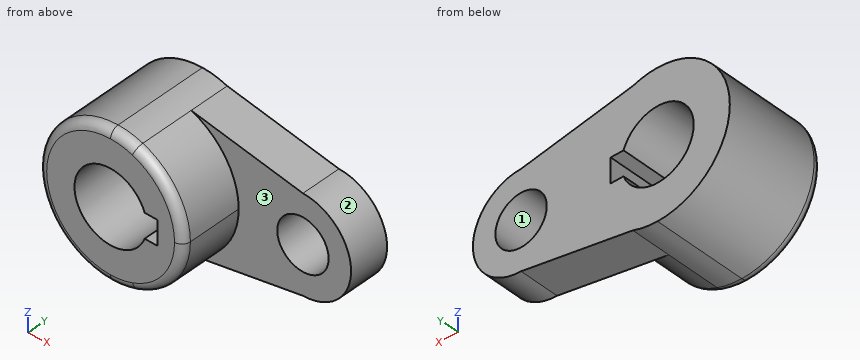
from build123d import *

# Parameters (mm, degrees)
F1_DEPTH = 40.2336
F0_R     = 10.16
F2_DEPTH = 15.7734
F3_R     = 3.302


with BuildPart() as f1:
    # F0 (on Front) → F1 (new body)
    with BuildSketch(Plane.XZ):
        with BuildLine():
            add(Edge.make_bspline(
                [(9.780704698, 26.8489932886), (6.5204697987, 27.4243288591), (3.2602348993, 27.9996644295), (0, 28.575)],
                knots=[44.8771660598, 44.8771660598, 44.8771660598, 44.8771660598, 54.8089978927, 54.8089978927, 54.8089978927, 54.8089978927], degree=3))
            ThreePointArc((0, 28.575), (-28.575, 0), (0, -28.575))
            add(Edge.make_bspline(
                [(9.780704698, -26.8489932886), (6.5204697987, -27.4243288591), (3.2602348993, -27.9996644295), (0, -28.575)],
                knots=[44.8771660598, 44.8771660598, 44.8771660598, 44.8771660598, 54.8089978927, 54.8089978927, 54.8089978927, 54.8089978927], degree=3))
            ThreePointArc((9.780704698, -26.8489932886), (23.4095521288, -16.3866864902), (28.575, 0))
            ThreePointArc((28.575, 0), (23.4095521288, 16.3866864902), (9.780704698, 26.8489932886))
        make_face()
        with BuildLine():
            ThreePointArc((13.4477648793, -4.826), (-14.2875, 0), (13.4477648793, 4.826))
            Line((13.4477648793, 4.826), (18.5293, 4.826))
            Line((18.5293, 4.826), (18.5293, -4.826))
            Line((18.5293, -4.826), (13.4477648793, -4.826))
        make_face(mode=Mode.SUBTRACT)
        with BuildLine():
            ThreePointArc((9.780704698, 26.8489932886), (4.9659159165, 28.1401901932), (0, 28.575))
            add(Edge.make_bspline(
                [(9.780704698, 26.8489932886), (6.5204697987, 27.4243288591), (3.2602348993, 27.9996644295), (0, 28.575)],
                knots=[44.8771660598, 44.8771660598, 44.8771660598, 44.8771660598, 54.8089978927, 54.8089978927, 54.8089978927, 54.8089978927], degree=3))
        make_face()
        with BuildLine():
            add(Edge.make_bspline(
                [(9.780704698, -26.8489932886), (6.5204697987, -27.4243288591), (3.2602348993, -27.9996644295), (0, -28.575)],
                knots=[44.8771660598, 44.8771660598, 44.8771660598, 44.8771660598, 54.8089978927, 54.8089978927, 54.8089978927, 54.8089978927], degree=3))
            ThreePointArc((0, -28.575), (4.9659159165, -28.1401901932), (9.780704698, -26.8489932886))
        make_face()
    extrude(amount=F1_DEPTH)

    # F0 (on Front) → F2 (join)
    with BuildSketch(Plane.XZ):
        with BuildLine():
            add(Edge.make_bspline(
                [(9.780704698, 26.8489932886), (6.5204697987, 27.4243288591), (3.2602348993, 27.9996644295), (0, 28.575)],
                knots=[44.8771660598, 44.8771660598, 44.8771660598, 44.8771660598, 54.8089978927, 54.8089978927, 54.8089978927, 54.8089978927], degree=3))
            ThreePointArc((0, 28.575), (-28.575, 0), (0, -28.575))
            add(Edge.make_bspline(
                [(9.780704698, -26.8489932886), (6.5204697987, -27.4243288591), (3.2602348993, -27.9996644295), (0, -28.575)],
                knots=[44.8771660598, 44.8771660598, 44.8771660598, 44.8771660598, 54.8089978927, 54.8089978927, 54.8089978927, 54.8089978927], degree=3))
            ThreePointArc((9.780704698, -26.8489932886), (23.4095521288, -16.3866864902), (28.575, 0))
            ThreePointArc((28.575, 0), (23.4095521288, 16.3866864902), (9.780704698, 26.8489932886))
        make_face()
        with BuildLine():
            ThreePointArc((13.4477648793, -4.826), (-14.2875, 0), (13.4477648793, 4.826))
            Line((13.4477648793, 4.826), (18.5293, 4.826))
            Line((18.5293, 4.826), (18.5293, -4.826))
            Line((18.5293, -4.826), (13.4477648793, -4.826))
        make_face(mode=Mode.SUBTRACT)
        with BuildLine():
            ThreePointArc((9.780704698, 26.8489932886), (4.9659159165, 28.1401901932), (0, 28.575))
            add(Edge.make_bspline(
                [(9.780704698, 26.8489932886), (6.5204697987, 27.4243288591), (3.2602348993, 27.9996644295), (0, 28.575)],
                knots=[44.8771660598, 44.8771660598, 44.8771660598, 44.8771660598, 54.8089978927, 54.8089978927, 54.8089978927, 54.8089978927], degree=3))
        make_face()
        with BuildLine():
            add(Edge.make_bspline(
                [(9.780704698, -26.8489932886), (6.5204697987, -27.4243288591), (3.2602348993, -27.9996644295), (0, -28.575)],
                knots=[44.8771660598, 44.8771660598, 44.8771660598, 44.8771660598, 54.8089978927, 54.8089978927, 54.8089978927, 54.8089978927], degree=3))
            ThreePointArc((0, -28.575), (4.9659159165, -28.1401901932), (9.780704698, -26.8489932886))
        make_face()
        with BuildLine():
            add(Edge.make_bspline(
                [(53.975, 19.05), (39.2435682327, 21.6496644295), (24.5121364653, 24.2493288591), (9.780704698, 26.8489932886)],
                knots=[0, 0, 0, 0, 44.8771660598, 44.8771660598, 44.8771660598, 44.8771660598], degree=3))
            ThreePointArc((9.780704698, 26.8489932886), (23.4095521288, 16.3866864902), (28.575, 0))
            ThreePointArc((28.575, 0), (23.4095521288, -16.3866864902), (9.780704698, -26.8489932886))
            add(Edge.make_bspline(
                [(53.975, -19.05), (39.2435682327, -21.6496644295), (24.5121364653, -24.2493288591), (9.780704698, -26.8489932886)],
                knots=[0, 0, 0, 0, 44.8771660598, 44.8771660598, 44.8771660598, 44.8771660598], degree=3))
            ThreePointArc((53.975, -19.05), (73.025, 0), (53.975, 19.05))
        make_face()
        with Locations((53.975, 0)):
            Circle(F0_R, mode=Mode.SUBTRACT)
    extrude(amount=F2_DEPTH)

    # F3
    f3_edges = [f1.edges().sort_by_distance(p)[0] for p in [
        (0, -40.2336, 28.575),
    ]]
    fillet(f3_edges, radius=F3_R)


solid = f1.part
Geometry: final body of the model. Coordinates: model frame, mm. Face numbers are marked on the shaded views. Coordinates: 2 decimals unless noted, no trailing zeros. Order: outer loops, then holes, each group sorted by start corner. A loop starts at its lowest first (then second) coordinate and runs counter-clockwise, first axis right, second up.
1) Draft query along X for the marked faces 1, 2 and 3. Return one class per face: released by +X, released by -X, zero draft, split by the parting line, or undercut.
Result sheet:
face 1: undercut
face 2: released by +X
face 3: zero draft
2) First-contact query: P1, Ø8, axis at x = 4.5, z = 5.5, coming from the -Y side; P2, Ø1, axis at y = -6.5, z = -18.5, coming from the -X side; P3, Ø1.5, axis at x = 32.5, y = -16, coming from the +Z side; P4, Ø2, axis at x = 35.5, z = -0.5, coming from the -Y side. Flat tips, straight axial feed; report the tip coordinate or a pass-through.
Result sheet:
P1: passes through
P2: stops at x = -22.19
P3: stops at z = 22.97
P4: stops at y = -15.77
3) Section B-B (x = 61.5). Return loops of the section in (y, z).
Result sheet:
outline: (-15.77, -17.5) - (0, -17.5) - (0, -6.83) - (-15.77, -6.83) - close; (-15.77, 6.83) - (0, 6.83) - (0, 17.5) - (-15.77, 17.5) - close
4) Ray query, probe 1 along X at (y, z) = (-20, 0) (1 decimal); probe 2 along X at (y, z) = (-11.5, 8); probe 3 along Y at (x, z) = (28, 8). Return the intervals inside material, ascending.
Result sheet:
probe 1: x = -28.6 to -14.3, 18.5 to 28.6
probe 2: x = -27.43 to -11.84, 11.84 to 47.71, 60.24 to 71.26
probe 3: y = -15.77 to 0
5) Section C-C (z = 1). Give the number of separate pieces and of enclosed holes in the cut face, then the cut area to 3 significant figures.
Result sheet:
separate pieces: 3
enclosed holes: 0
area: 1,360 mm2
